Geometry check sheet. Reference: the model listing, model coordinates, mm. Face numbers are marked on the shaded views. Coordinates: 2 decimals unless noted, no trailing zeros. Order: outer loops, then holes, each group sorted by start corner. A loop starts at its lowest first (then second) coordinate and runs counter-clockwise, first axis right, second up. Notation, with made-up numbers: M 55,-11 L 87,-11 A27 cw 87,18 Z; hole C 69.5,46.5 d3. An arc over 180 degrees is marked long. Use CSV: the item, a comma, the result in double quotes. Start each with the question number.
```python
from build123d import *

# Parameters (mm, degrees)
SKETCH1_W           = 42
SKETCH1_H           = 13.15
BOSS_EXTRUDE1_DEPTH = 1.3
BOSS_EXTRUDE3_START = -5.1
BOSS_EXTRUDE3_DEPTH = 22.35
BOSS_EXTRUDE4_DEPTH = 1.5


with BuildPart() as part:
    # Sketch1 → Boss-Extrude1 (new body)
    with BuildSketch(Plane(origin=(0, 0, 0), x_dir=(1, 0, 0), z_dir=(0, 1, 0))):
        with Locations((21, 6.575)):
            Rectangle(SKETCH1_W, SKETCH1_H)
    extrude(amount=BOSS_EXTRUDE1_DEPTH)

    # Sketch3 → Boss-Extrude3 (add)
    with BuildSketch(Plane.ZY.offset(BOSS_EXTRUDE3_START)):
        Polygon((-13.15, 1.3), (-10.15, 1.3), (-10.15, 3.032050808), align=None)
    extrude(amount=-BOSS_EXTRUDE3_DEPTH)

    # Sketch4 → Boss-Extrude4 (add)
    with BuildSketch(Plane(origin=(0, 1.3, 0), x_dir=(1, 0, 0), z_dir=(0, 1, 0))):
        Polygon((40.9, 1.1), (40.9, 12.05), (28.55, 12.05), (28.55, 11.25), (40.1, 11.25), (40.1, 1.9), (1.1, 1.9), (1.1, 1.1), align=None)
    extrude(amount=BOSS_EXTRUDE4_DEPTH)


solid = part.part
```
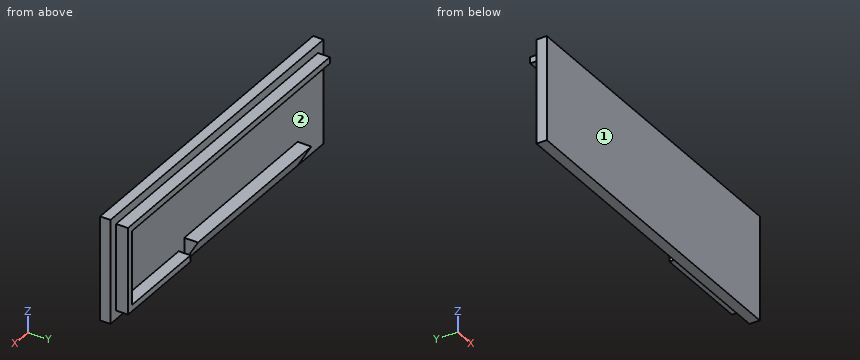
1) Draft check along Z on the marked faces 1 and 2. Enter one of: +Z half, -Z half, draft (parallel to the pull), parting line (faces both ways), or undercut.
2) Gauge pin test, flat ends, axial feed: P1, Ø5, axis at x = 34, z = -8, coming from the +Y side; P2, Ø1.2, axis at x = 35.5, y = 2, coming from the +Z side; P3, Ø1.5, axis at y = 2, z = -11.5, coming from the -X side; P4, Ø0.9, axis at y = 2, z = -1.5, coming from the -X side. Record the tip position at first contact, or that the pin passes through.
3) Material ranges on line 1 along Z through (x, y) = (35, 1.75); line 2 along Y through (x, z) = (37.5, -1.5); line 3 along X through (y, z) = (2.15, -4.25), recorded low to high.
4) Section check B-B on x = 3. Record the boundary of the cut face in (y, z).
5) Section check C-C on z = -1.5. Record the boundary of the cut face in (x, y).
6) Section check A-A on y = 2. Record the boundary of the cut face in (x, z), then the cut area to 3 significant figures.
7) Section check D-D on x = 13. Record the boundary of the cut face in (y, z).
Results are:
1,face 1,"draft"
1,face 2,"undercut"
2,P1,"stops at y = 1.3"
2,P2,"stops at z = -1.1"
2,P3,"stops at x = 0"
2,P4,"stops at x = 1.1"
3,line 1,"z = -12.05 to -11.25, -1.9 to -1.1"
3,line 2,"y = 0 to 2.8"
3,line 3,"x = 40.1 to 40.9"
4,outline,"M 0,-13.15 L 1.3,-13.15 L 1.3,-1.9 L 2.8,-1.9 L 2.8,-1.1 L 1.3,-1.1 L 1.3,0 L 0,0 Z"
5,outline,"M 0,0 L 42,0 L 42,1.3 L 40.9,1.3 L 40.9,2.8 L 1.1,2.8 L 1.1,1.3 L 0,1.3 Z"
6,outline,"M 1.1,-1.9 L 40.1,-1.9 L 40.1,-11.25 L 28.55,-11.25 L 28.55,-12.05 L 40.9,-12.05 L 40.9,-1.1 L 1.1,-1.1 Z; M 5.1,-11.94 L 27.45,-11.94 L 27.45,-10.15 L 5.1,-10.15 Z"
6,area,"89.2 mm²"
7,outline,"M 0,-13.15 L 1.3,-13.15 L 3.03,-10.15 L 1.3,-10.15 L 1.3,-1.9 L 2.8,-1.9 L 2.8,-1.1 L 1.3,-1.1 L 1.3,0 L 0,0 Z"
